For this review, use the dimensioned drawing (mm, ordinates from the lowest corner) and the shaded views. A direction names the side the tool comes from. Give positions to 0.01 mm unless a question says otherwise; leave off trailing zeros. Order: outer loops, then holes, each group sorted by start corner. A loop starts at its lowest first (then second) coordinate and runs counter-clockwise, first axis right, second up. Notation, with made-up numbers: (-1, -4) - (11, -4) arc R12 cw to (11, 19) - close; hole circle Ø8 at (28, -24.5). An arc over 180 degrees is marked (long way). Use a Markdown table: item, result. Add a question column.
1) We need section C-C on x = 4. Write out the cut boundary in (y, z).
2) Wall thickness on L1, parallel to Z at x = 3, y = 6.5; L2, parallel to X at y = 3.75, z = 12: over which ranges is each line inside the solid? List them lowest first.
3) We need section B-B on y = 1.5. Write out the cut boundary in (x, z), then the cut area to 3 significant figures.
4) We need section A-A on x = 7. Write out the cut boundary in (y, z), then the cut area to 3 significant figures.
5) Clearance check with flat-ended pins moving along their axes: P1, Ø3, axis at x = 5.5, z = 4, coming from the +Y side; P2, Ø1.5, axis at y = 2.5, z = 22, coming from the -X side; P3, Ø2, axis at y = 1.5, z = 6.5, coming from the +X side. State where each tip first meets the part, or that it passes through.
6) Machinability: for the marked faces 1, 2 and 3, which of the approach directions +Z, -Z, +X, -X, +Y, -Y give a long, thin tool a straight path to every point of the face, cutting with its end or side? Answer none if there is none.
7) Mouldability with a two-part tool opening along Z and no side actions: class the marked faces 4, 5 and 6 as released by +Z, released by -Z, zero draft, split by the parting line, or undercut.
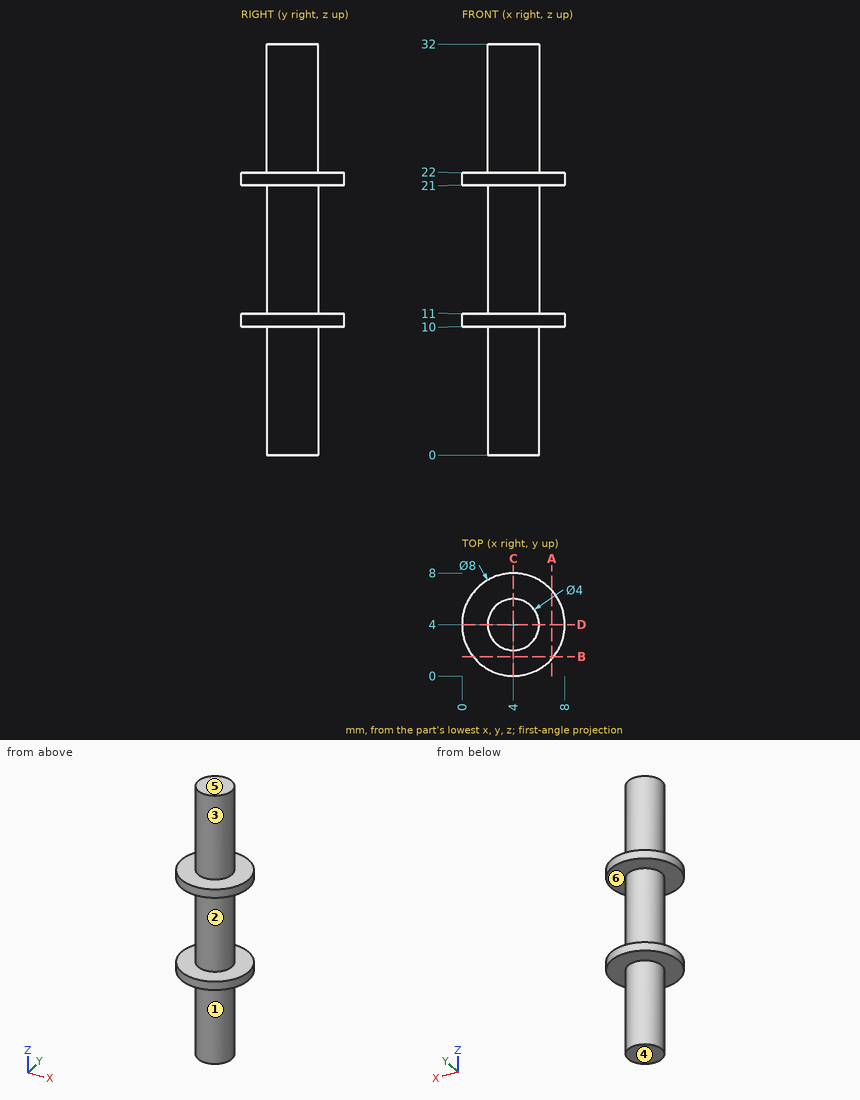
Checked values:
| question | item | result |
|---|---|---|
| 1 | outline | (0, 10) - (2, 10) - (2, 0) - (6, 0) - (6, 10) - (8, 10) - (8, 11) - (6, 11) - (6, 21) - (8, 21) - (8, 22) - (6, 22) - (6, 32) - (2, 32) - (2, 22) - (0, 22) - (0, 21) - (2, 21) - (2, 11) - (0, 11) - close |
| 2 | L1 | 10 to 11, 21 to 22 |
| 2 | L2 | 2.02 to 5.98 |
| 3 | outline | (0.88, 10) - (7.12, 10) - (7.12, 11) - (0.88, 11) - close; (0.88, 21) - (7.12, 21) - (7.12, 22) - (0.88, 22) - close |
| 3 | area | 12.5 mm² |
| 4 | outline | (1.35, 10) - (6.65, 10) - (6.65, 11) - (1.35, 11) - close; (1.35, 21) - (6.65, 21) - (6.65, 22) - (1.35, 22) - close |
| 4 | area | 10.6 mm² |
| 5 | P1 | y = 6 |
| 5 | P2 | x = 0.07 |
| 5 | P3 | x = 5.32 |
| 6 | face 1 | -Z |
| 6 | face 2 | none |
| 6 | face 3 | +Z |
| 7 | face 4 | released by -Z |
| 7 | face 5 | released by +Z |
| 7 | face 6 | undercut |
